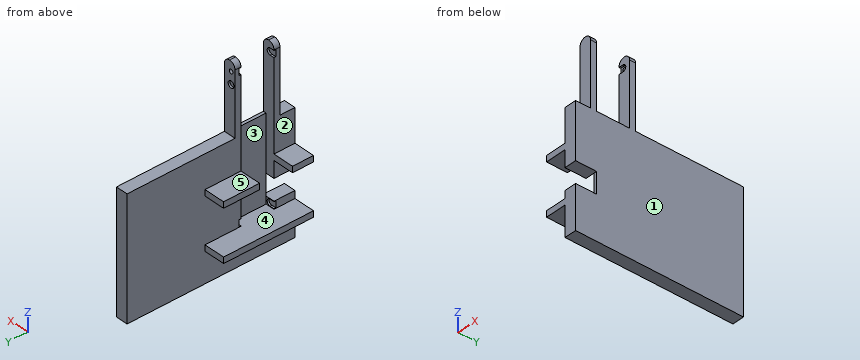
```python
from build123d import *

# Parameters (mm, degrees)
SKETCH_1_W          = 20
SKETCH_1_H          = 280
EXTRUDE_1_DEPTH     = 200
SKETCH_2_W          = 35
SKETCH_2_H          = 35
CUT_EXTRUDE_1_DEPTH = 245.948974278
SKETCH_4_W          = 35
SKETCH_4_H          = 10
EXTRUDE_2_DEPTH     = 150
SKETCH_5_W          = 35
SKETCH_5_H          = 55
CUT_EXTRUDE_3_DEPTH = 24
CUT_EXTRUDE_4_REACH = 250.244
SKETCH_6_W          = 15
SKETCH_6_H          = 55
CUT_EXTRUDE_START   = -3
CUT_EXTRUDE_5_DEPTH = 61
SKETCH_9_W          = 20
SKETCH_9_H          = 10
EXTRUDE_3_DEPTH     = 115
SKETCH_10_R         = 3.5
CUT_EXTRUDE_7_DEPTH = 20
SKETCH_11_R         = 5.5
CUT_EXTRUDE_8_DEPTH = 3
FILLET_1_R          = 10


with BuildPart() as part:
    # 草图1 → 凸台-拉伸1 (new body)
    with BuildSketch(Plane.XY):
        Rectangle(SKETCH_1_W, SKETCH_1_H)
    extrude(amount=EXTRUDE_1_DEPTH)

    # 草图2 → 切除-拉伸1 (cut, through all)
    with BuildSketch(Plane.ZY.offset(10)):
        with Locations((89.937894672, -122.5)):
            Rectangle(SKETCH_2_W, SKETCH_2_H)
    extrude(amount=-CUT_EXTRUDE_1_DEPTH, mode=Mode.SUBTRACT)

    # 草图4 → 凸台-拉伸2 (add)
    with BuildSketch(Plane.XZ.offset(140)):
        with Locations((-27.5, 54.987894672)):
            Rectangle(SKETCH_4_W, SKETCH_4_H)
        with Locations((-27.5, 139.987894672)):
            Rectangle(SKETCH_4_W, SKETCH_4_H)
    extrude(amount=-EXTRUDE_2_DEPTH)

    # 草图5 → 切除-拉伸3 (cut)
    with BuildSketch(Plane.XY.offset(144.987894672)):
        with Locations((-27.5, -77.5)):
            Rectangle(SKETCH_5_W, SKETCH_5_H)
    extrude(amount=-CUT_EXTRUDE_3_DEPTH, mode=Mode.SUBTRACT)

    # 切除-拉伸4: up to this face of the body (flat: up to its plane)
    cut_extrude_4_end = Plane(part.part.faces().sort_by_distance((-27.5, -65, 59.987894672))[0])
    # 草图6 → 切除-拉伸4 (cut, up to the picked face)
    with BuildSketch(Plane.XY.offset(200), mode=Mode.PRIVATE) as cut_extrude_4_sk1:
        with Locations((-2.5, -77.5)):
            Rectangle(SKETCH_6_W, SKETCH_6_H)
    cut_extrude_4_tool1 = split(extrude(cut_extrude_4_sk1.sketch, amount=-CUT_EXTRUDE_4_REACH, mode=Mode.PRIVATE), bisect_by=cut_extrude_4_end, keep=Keep.BOTH, mode=Mode.PRIVATE)
    add(cut_extrude_4_tool1.solids().sort_by(Axis((-2.5, -77.5, 200), (0, 0, -1)))[0], mode=Mode.SUBTRACT)

    # 草图7 → 切除-拉伸5 (cut)
    with BuildSketch(Plane(origin=(0, -105, 0), x_dir=(1, 0, 0), z_dir=(0, 1, 0)).offset(CUT_EXTRUDE_START)):
        with BuildLine():
            Line((-2.661336035, -71.712894672), (-10, -71.712894672))
            Line((-10, -71.712894672), (-10, -60.712894672))
            Line((-10, -60.712894672), (-2.661336035, -60.712894672))
            ThreePointArc((-2.661336035, -60.712894672), (2.838663965, -66.212894672), (-2.661336035, -71.712894672))
        make_face()
    cut_extrude_5 = extrude(amount=CUT_EXTRUDE_5_DEPTH, mode=Mode.SUBTRACT)

    # 草图9 → 凸台-拉伸3 (add)
    with BuildSketch(Plane.XY.offset(200)):
        with Locations((0, -110)):
            Rectangle(SKETCH_9_W, SKETCH_9_H)
        with Locations((0, -45)):
            Rectangle(SKETCH_9_W, SKETCH_9_H)
    extrude(amount=EXTRUDE_3_DEPTH)

    # 镜向1: 切除-拉伸5 across plane
    add(cut_extrude_5.mirror(Plane(origin=(0, 0, 182.493947336), x_dir=(1, 0, 0), z_dir=(0, 0, -1))), mode=Mode.SUBTRACT)

    # 草图10 → 切除-拉伸7 (cut)
    with BuildSketch(Plane(origin=(0, -40, 0), x_dir=(1, 0, 0), z_dir=(0, 1, 0))):
        with Locations(Location((-2.661336035, -298.775, 0), (0, 0, 270))):
            Circle(SKETCH_10_R)
    extrude(amount=-CUT_EXTRUDE_7_DEPTH, mode=Mode.SUBTRACT)

    # 草图11 → 切除-拉伸8 (cut)
    with BuildSketch(Plane(origin=(0, -40, 0), x_dir=(1, 0, 0), z_dir=(0, 1, 0))):
        with Locations(Location((-2.5, -278.775, 0), (0, 0, 270))):
            Circle(SKETCH_11_R)
    extrude(amount=-CUT_EXTRUDE_8_DEPTH, mode=Mode.SUBTRACT)

    # 圆角1
    fillet_1_edges = [part.edges().sort_by_distance(p)[0] for p in [
        (10, -45, 315),
        (10, -110, 315),
        (-10, -45, 315),
        (-10, -110, 315),
    ]]
    fillet(fillet_1_edges, radius=FILLET_1_R - 0.0001)  # a hair under: the kernel refuses the full size


solid = part.part
```
CAD build for the part. Positions are in the model's coordinates, mm. Face numbers are marked on the shaded views. A direction names the side the tool comes from. Coordinates: 2 decimals unless noted, no trailing zeros. Write each loop counter-clockwise with the first axis right and the second up, starting at its lowest first coordinate (ties: lowest second). Pieces come first, ordered by that corner, then holes. Notation, with made-up numbers: (-22, -23.75) -> (-16, -23.75) arc R19 cw to (-16, -11.75) -> close; hole circle Ø8 at (-34.75, 75). An arc over 180 degrees is marked (long way). Return JSON: item names as keys, results as strings. Group by question number.
Q1. Pull direction Y, two halves, no side cores. Call the marked faces 4 and 5: released by +Y, released by -Y, zero draft, split by the parting line, or undercut.
Q2. Cut at A-A, the plane x = -19. Give the cut face in (y, z), then the cut area to 3 significant figures.
Q3. Drill centre lines: line 1 (Z direction, x = -18, y = 1.5); line 2 (Z direction, x = -4, y = -116); line 3 (Y direction, x = -2, z = 238.5). Where is each one in solid material? Low to high.
Q4. Which spindle directions (+Z, -Z, +X, -X, +Y, -Y) get a long thin tool onto all of the face, cutting with end or side? Do the marked faces 1, 2 and 3. Say none if no direction does.
Q5. Flat gauge pins, fed straight in: pin 1 (2.5 mm diameter, centred on x = -6, y = -106, fed in from +Z); pin 2 (25 mm diameter, centred on x = -24, y = -65, fed in from +Z); pin 3 (6 mm diameter, centred on y = -115.5, z = 67, fed in from -X). Where does each tip first touch, or does it go through?
Q6. Cut at C-C, the plane y = -75.5. Give the cut face in (x, z), then the cut area to 3 significant figures.
Q7. Cut at D-D, the plane z = 46.5. Give the cut face in (x, y).
Q8. Cut at B-B, the plane z = 231. Give the cut face in (x, y), then the cut area to 3 significant figures.
Returned:
{
 "1": {"face 4": "undercut", "face 5": "zero draft"},
 "2": {"outline": "(-140, 49.99) -> (10, 49.99) -> (10, 59.99) -> (-140, 59.99) -> close; (-140, 134.99) -> (-105, 134.99) -> (-105, 144.99) -> (-140, 144.99) -> close; (-50, 134.99) -> (10, 134.99) -> (10, 144.99) -> (-50, 144.99) -> close", "area": "2,450 mm2"},
 "3": {"line 1": "z = 49.99 to 59.99, 134.99 to 144.99", "line 2": "z = 0 to 72.44, 107.44 to 200", "line 3": "y = -115 to -105, -50 to -40"},
 "4": {"face 1": "+Z, -Z, +X, +Y, -Y", "face 2": "+Z, -X, +Y, -Y", "face 3": "+Z, -X"},
 "5": {"pin 1": "stops at z = 313.8", "pin 2": "stops at z = 59.99", "pin 3": "stops at x = -10"},
 "6": {"outline": "(-45, 49.99) -> (-10, 49.99) -> (-10, 0) -> (10, 0) -> (10, 200) -> (5, 200) -> (5, 59.99) -> (-45, 59.99) -> close", "area": "2,250 mm2"},
 "7": {"outline": "(-10, -140) -> (10, -140) -> (10, 140) -> (-10, 140) -> close"},
 "8": {"outline": "(-10, -115) -> (10, -115) -> (10, -105) -> (-10, -105) -> close; (-10, -50) -> (10, -50) -> (10, -40) -> (-10, -40) -> close", "area": "400 mm2"}
}
